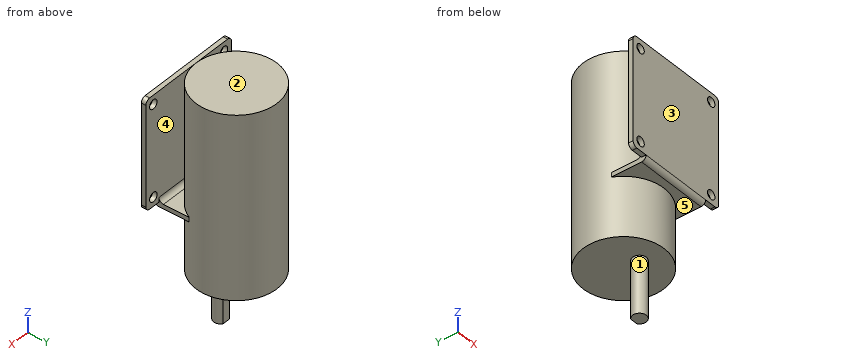
Autodesk Inventor part; units mm, degrees
ref_plane "Plan de construction1" through (0, 0, 26) normal (0, 0, -1) x (-1, 0, 0)
ref_plane "YZ Plane" through (0, 0, 0) normal (1, 0, 0) x (0, 1, 0)
ref_plane "XZ Plane" through (0, 0, 0) normal (0, 1, 0) x (-1, 0, 0)
sketch "Esquisse1" plane through (0, 0, 0) normal (0, 0, 1) x (1, 0, 0)
  arc A0 (-1.6583, -4.5) -> (1.6583, -4.5) centre (0, -7) ccw
  line L0 (1.6583, -4.5) -> (-1.6583, -4.5)
  point P0 (0, 0)
  dimension "d2" = 6
  dimension "d4" = 7
  dimension "d11" = 0.5
extrude "Extrusion1" add sketch "Esquisse1" against normal blind 25
sketch "Esquisse2" plane through (0, -7, 0) normal (0, 0, 1) x (1, 0, 0)
  circle A0 centre (0, 7) radius 17.75
  dimension "d8" = 35.5
extrude "Extrusion2" add sketch "Esquisse2" along normal blind 80
ref_plane "Plan de construction1" through (0, 0, 26) normal (0, 0, -1) x (-1, 0, 0)
sketch "Esquisse3" plane through (0, 0, 26) normal (0, 0, -1) x (-1, 0, 0)
  circle A0 centre (0, 0) radius 17.75
  line L0 (1.6583, -4.5) -> (-1.6583, -4.5)
  arc A1 (-1.6583, -4.5) -> (1.6583, -4.5) centre (0, -7) ccw
  line L1 (-16, -7.6852) -> (-16, -21)
  line L2 (-16, -21) -> (0, -21)
  line L3 (16, -7.6852) -> (16, -21)
  line L4 (16, -21) -> (0, -21)
  arc A2 (-16, -7.6852) -> (16, -7.6852) centre (0, 0) ccw
  circle A3 centre (0, 0) radius 17.75
  line L5 (-3, -7) -> (0, -7)
  line L6 (0, -4.5) -> (0, -7)
  dimension "d14" = 16
extrude "Extrusion3" add sketch "Esquisse3" against normal blind 2 contours A0 L3 L4 L2 L1
sketch "Esquisse4" plane through (0, 0, 28) normal (0, 0, 1) x (1, 0, 0)
  line L0 (-23, -21) -> (23, -21)
  line L1 (23, -21) -> (23, -23)
  line L2 (23, -23) -> (-23, -23)
  line L3 (-23, -23) -> (-23, -21)
  point P0 (0, 0)
  dimension "d18" = 2
  dimension "d19" = 46
extrude "Extrusion4" add sketch "Esquisse4" along normal blind 48
fillet "Congé1" radius 2 4 edges at (-23, -22, 28) (-23, -22, 76) (23, -22, 76) (23, -22, 28)
sketch "Esquisse5" plane through (16, -21, 26) normal (1, 0, 0) x (0, 0, -1)
  arc A0 (-2, -2) -> (0, 0) centre (-2, 0) ccw
  line L0 (-2, 0) -> (-2, -2)
  line L1 (-2, -2) -> (-2, 0)
  line L2 (-2, 0) -> (0, 0)
  line L3 (0, 0) -> (-2, 0)
  point P0 (26, 21)
extrude "Extrusion5" add sketch "Esquisse5" against normal blind 32
fillet "Congé2" radius 2 1 edges at (0, -21, 28)
sketch "Esquisse6" plane through (-21, -21, 28) normal (0, 1, 0) x (1, 0, 0)
  line L0 (40, -4) -> (2, -4)
  line L1 (2, -4) -> (2, -44)
  line L2 (2, -44) -> (40, -44)
  line L3 (40, -44) -> (40, -4)
  line L4 (44, -2) -> (44, -46)
  line L5 (42, 0) -> (37, 0)
  line L6 (42, -48) -> (0, -48)
  line L7 (-2, -2) -> (-2, -46)
  point P0 (21, 28)
  dimension "d28" = 4
  dimension "d29" = 4
  dimension "d30" = 4
  dimension "d31" = 4
hole "Perçage1" at (-19, -21, 32) at (-19, -21, 72) at (19, -21, 72) at (19, -21, 32) direction (0, -1, 0) diameter 4 end through all
properties part number "Moteur"
Geometry check sheet. Reference: the model listing, model coordinates, mm. Face numbers are marked on the shaded views. A direction names the side the tool comes from. Give positions to 0.01 mm unless a question says otherwise; leave off trailing zeros. Order: outer loops, then holes, each group sorted by start corner. A loop starts at its lowest first (then second) coordinate and runs counter-clockwise, first axis right, second up. Notation, with made-up numbers: (68.25, 61.5) -> (97.25, 61.5) arc R24 cw to (97.25, 94.5) -> close; hole circle Ø3 at (70.25, 63.25). An arc over 180 degrees is marked (long way). Write each question's results on one line, items separated by ' | '. Start each with the question number.
(1) Scan lines: line 1 (Z direction, x = -19, y = -22); line 2 (X direction, y = -22, z = 72); line 3 (Z direction, x = 11.5, y = -10.5). Record each from-to range of solid material in increasing order.
(2) Sectioned sample at B-B (z = 32). Enter the section's corners in (x, y), plus the area to 3 significant figures.
(3) Mould release check, pull along Y, two halves, no side actions. Record for the marked faces 3, 4 and 5: pulls with the +Y half, pulls with the -Y half, needs draft (parallel to the pull), parting line crosses it, or undercut.
(4) Access from +Z, -Z, +X, -X, +Y, -Y to the whole of each face (thin tool, end or side, straight path). Record for the marked faces 1 and 2.
(5) Sectioned sample at A-A (x = -19). Enter the section's corners in (y, z), plus the area to 3 significant figures.
(6) Gauge pin test, flat ends, axial feed: P1, Ø2.5, axis at x = 0.5, z = -13, coming from the +Y side; P2, Ø0.6, axis at x = -4.5, y = -22.5, coming from the +Z side; P3, Ø4, axis at x = 8.5, y = -4, coming from the -Z side. Record the tip position at first contact, or that the pin passes through.
(7) Sectioned sample at C-C (x = 11.5). Enter the section's corners in (y, z).
(8) Sectioned sample at D-D (y = 2). Enter the section's corners in (x, z), plus the area to 3 significant figures.
Answer below:
1) line 1: 28 to 30, 34 to 70, 74 to 76 | line 2: -23 to -21, -17 to 17, 21 to 23 | line 3: 0 to 80
2) outline: (-23, -23) -> (-21, -23) -> (-21, -21) -> (-23, -21) -> close; circle Ø35.5 at (0, 0); (-17, -23) -> (17, -23) -> (17, -21) -> (-17, -21) -> close; (21, -23) -> (23, -23) -> (23, -21) -> (21, -21) -> close | area: 1,070 mm2
3) face 3: pulls with the -Y half | face 4: undercut | face 5: needs draft
4) face 1: -Z | face 2: +Z, +X, -X, +Y, -Y
5) outline: (-23, 28) -> (-21, 28) -> (-21, 30) -> (-23, 30) -> close; (-23, 34) -> (-21, 34) -> (-21, 70) -> (-23, 70) -> close; (-23, 74) -> (-21, 74) -> (-21, 76) -> (-23, 76) -> close | area: 80.0 mm2
6) P1: y = -4.5 | P2: z = 76 | P3: z = 0
7) outline: (-23, 28) arc R2 ccw to (-21, 26) -> (-13.52, 26) -> (-13.52, 0) -> (13.52, 0) -> (13.52, 80) -> (-13.52, 80) -> (-13.52, 28) -> (-19, 28) arc R2 cw to (-21, 30) -> (-21, 76) -> (-23, 76) -> close
8) outline: (-17.64, 0) -> (17.64, 0) -> (17.64, 80) -> (-17.64, 80) -> close | area: 2,820 mm2
